from build123d import *

# Parameters (mm, degrees)
F0_W      = 120
F0_H      = 60
F1_DEPTH  = 20
F2_W      = 20
F2_H      = 2
F3_DEPTH  = 25.5
F4_W      = 20
F4_H      = 2
F3_FACE_W = 20
F3_FACE_H = 2
F5_ANGLE  = 180


# Not quite as in the source:
# - a feature names something its author has since deleted; it is built from what else it names


with BuildPart() as f1:
    # F0 (on Top) → F1 (new body)
    with BuildSketch(Plane.XY):
        Rectangle(F0_W, F0_H)
    extrude(amount=F1_DEPTH)

    # F2 (on face) → F3 (join)
    with BuildSketch(Plane(origin=(0, 0, 0), x_dir=(1, 0, 0), z_dir=(0, 0, -1))):
        with Locations((-39.2824916542, 26.5)):
            Rectangle(F2_W, F2_H)
        with Locations((-39.2824916542, -26.5)):
            Rectangle(F2_W, F2_H)
        with Locations((0.8980135992, 26.5)):
            Rectangle(F2_W, F2_H)
        with Locations((0.8980135992, -26.5)):
            Rectangle(F2_W, F2_H)
        with Locations((45.2481971681, 26.5)):
            Rectangle(F2_W, F2_H)
        with Locations((45.2481971681, -26.5)):
            Rectangle(F2_W, F2_H)
    extrude(amount=F3_DEPTH)

    # F4 (on face) + F3_face (on face) → F5 (revolve)
    with BuildSketch(Plane(origin=(0, 0, -25.5), x_dir=(1, 0, 0), z_dir=(0, 0, -1))):
        with Locations((-39.2824916542, 26.5)):
            Rectangle(F4_W, F4_H)
    with BuildSketch(Plane(origin=(-39.2824916542, -26.5, -25.5), x_dir=(1, 0, 0), z_dir=(0, 0, -1))):
        with Locations((40.1805052534, 0)):
            Rectangle(F3_FACE_W, F3_FACE_H)
        with Locations((84.5306888223, 0)):
            Rectangle(F3_FACE_W, F3_FACE_H)
    revolve(axis=Axis((1.9900724292, 0, -25.5), (1, 0, 0)), revolution_arc=F5_ANGLE)


solid = f1.part
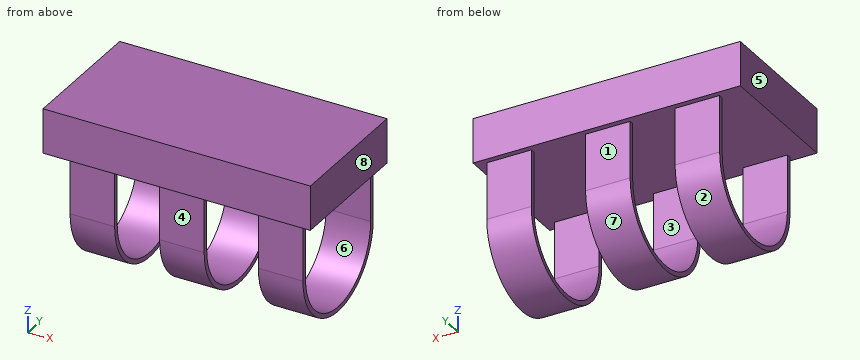
Here's how the part is built. I have some questions about the finished solid (model axes, mm). Face numbers are marked on the shaded views. A direction names the side the tool comes from. Give positions to 0.01 mm unless a question says otherwise; leave off trailing zeros. Order: outer loops, then holes, each group sorted by start corner. A loop starts at its lowest first (then second) coordinate and runs counter-clockwise, first axis right, second up. Notation, with made-up numbers: M -2.75,-7.5 L 56.25,-7.5 A11 cw 56.25,12.5 Z; hole C 27.25,10 d4. An arc over 180 degrees is marked long. Answer as a JSON object with one key per item and string values. Group by question number.
1) Suppose I cut it at D-D, the plane y = -23. Write out the boundary of the cut face in (x, z).
2) Suppose I cut it at B-B, the plane x = -41.5. Write out the boundary of the cut face in (y, z).
3) I'm going to push flat-ended pins straight in: pin 1 Ø22 at (x, z) = (47, -15.5) entering from -Y; pin 2 Ø10 at (x, y) = (-28, 5.5) entering from -Z; pin 3 Ø10 at (x, z) = (49, -14) entering from +Y; pin 4 Ø16 at (y, z) = (13.5, -34.5) entering from -X. Where does each tip first touch, or does it pass through?
4) Suppose I cut it at C-C, the plane z = -7. Write out the boundary of the cut face in (x, y), plus the area to 3 significant figures.
5) We'd pull the mould along Z, two halves only. Please class the marked faces 6, 7 and 8: pulls with the +Z half, pulls with the -Z half, needs draft (parallel to the pull), parting line crosses it, or undercut.
6) On a 3-axis mill with a long thin cutter (end or side, diameter ignored), from which of +Z, -Z, +X, -X, +Y, -Y can I reach the whole of each face in a straight line? I mean the marked faces 1, 2, 3, 4 and 5. Say none if no direction works.
7) Please list where these lines run through material, in increasing order: L1, parallel to Y at x = -2, z = -0.5; L2, parallel to Z at x = -24, y = -14.5; L3, parallel to Z at x = 7.5, y = 19. Write a range as [from, to].
8) Suppose I cut it at A-A, the plane y = 0. Write out the boundary of the cut face in (x, z), plus the area to 3 significant figures.
Results found:
{
 "1": {"outline": "M -60,0 L 60,0 L 60,20 L -60,20 Z; M -49.28,-40.57 L -29.28,-40.57 L -29.28,-36.51 L -49.28,-36.51 Z; M -9.1,-40.57 L 10.9,-40.57 L 10.9,-36.51 L -9.1,-36.51 Z; M 35.25,-40.57 L 55.25,-40.57 L 55.25,-36.51 L 35.25,-36.51 Z"},
 "2": {"outline": "M -30,0 L -27.5,0 L -27.5,-25.5 A27.5 ccw 27.5,-25.5 L 27.5,0 L 30,0 L 30,20 L -30,20 Z; hole M -25.5,-25.5 A25.5 ccw 25.5,-25.5 L 25.5,0 L -25.5,0 Z"},
 "3": {"pin 1": "y = -27.5", "pin 2": "z = -52.99", "pin 3": "y = 27.5", "pin 4": "through"},
 "4": {"outline": "M -49.28,-27.5 L -29.28,-27.5 L -29.28,-25.5 L -49.28,-25.5 Z; M -49.28,25.5 L -29.28,25.5 L -29.28,27.5 L -49.28,27.5 Z; M -9.1,-27.5 L 10.9,-27.5 L 10.9,-25.5 L -9.1,-25.5 Z; M -9.1,25.5 L 10.9,25.5 L 10.9,27.5 L -9.1,27.5 Z; M 35.25,-27.5 L 55.25,-27.5 L 55.25,-25.5 L 35.25,-25.5 Z; M 35.25,25.5 L 55.25,25.5 L 55.25,27.5 L 35.25,27.5 Z", "area": "240 mm²"},
 "5": {"face 6": "undercut", "face 7": "pulls with the -Z half", "face 8": "needs draft"},
 "6": {"face 1": "-Z, +X, -X, +Y", "face 2": "-Z, +X, -X", "face 3": "+X, -X", "face 4": "-Z, +X, -X, -Y", "face 5": "+Z, -Z, -X, +Y, -Y"},
 "7": {"L1": "[-27.5, -25.5], [25.5, 27.5]", "L2": "[0, 20]", "L3": "[-45.38, -42.51], [0, 20]"},
 "8": {"outline": "M -60,0 L 60,0 L 60,20 L -60,20 Z; M -49.28,-53 L -29.28,-53 L -29.28,-51 L -49.28,-51 Z; M -9.1,-53 L 10.9,-53 L 10.9,-51 L -9.1,-51 Z; M 35.25,-53 L 55.25,-53 L 55.25,-51 L 35.25,-51 Z", "area": "2,520 mm²"}
}
